Geometry: see drawing. Coordinates: mm, zero at the bounding-box minimum. A direction names the side the tool comes from. Coordinates: 2 decimals unless noted, no trailing zeros. Loops run counter-clockwise (first coordinate to the right, second up) from the corner with the lowest first, then second, coordinate; pieces in that order, holes last.
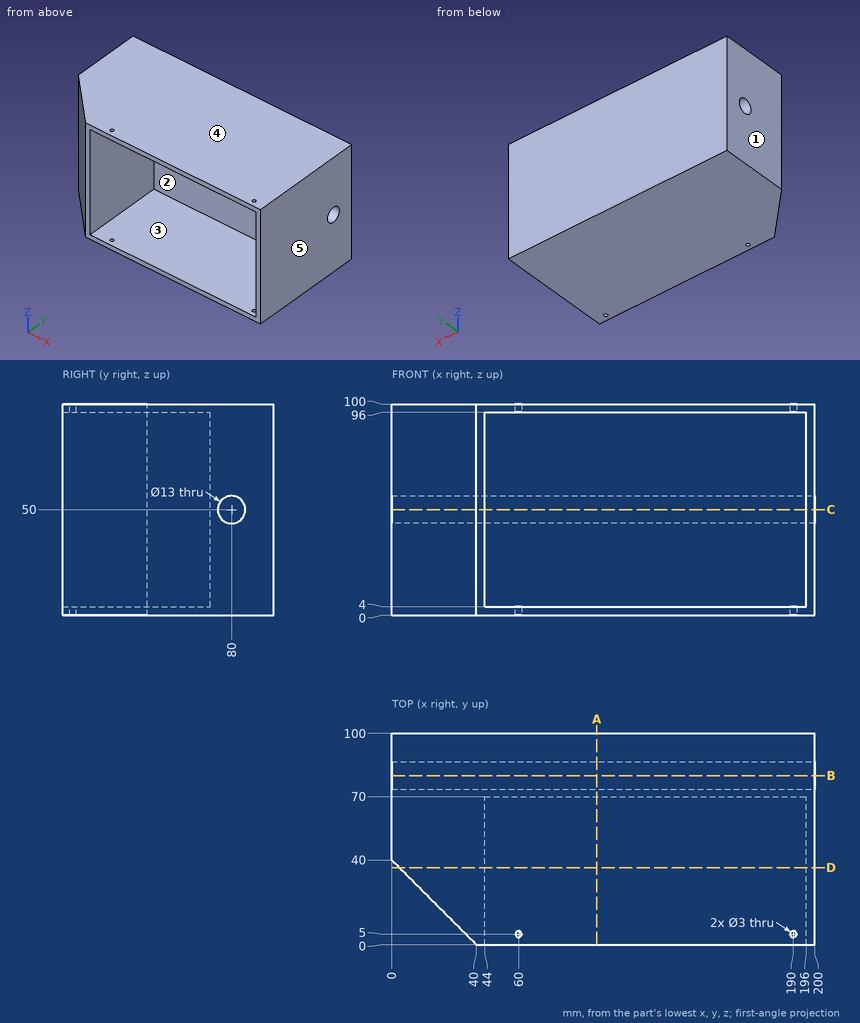
Item 1: Reachability of the marked faces 1 and 2 from +Z, -Z, +X, -X, +Y, -Y: full face, straight path, thin tool, end or side. Return the list, or none.
Result:
face 1: +Z, -Z, -X, +Y, -Y
face 2: -Y
Item 2: Section query A-A (x = 97). Output: boundary loops of the cut face in (y, z), then the cut area to 3 significant figures.
Result:
outline: (0, 0) - (100, 0) - (100, 100) - (0, 100) - (0, 96) - (70, 96) - (70, 4) - (0, 4) - close; hole circle Ø13 at (80, 50)
area: 3,430 mm2
Item 3: Line query: L1, parallel to Z at x = 54.5, y = 20.5; L2, parallel to X at y = 47.5, z = 79; L3, parallel to Y at x = 60, z = 98. Output: solid intervals per line, ascending.
Result:
L1: z = 0 to 4, 96 to 100
L2: x = 0 to 44, 196 to 200
L3: y = 0 to 3.5, 6.5 to 100
Item 4: Contact query for flat-ended pins moving along their axis: P1, Ø10, axis at y = 34.5, z = 59, coming from the -X side; P2, Ø3, axis at x = 147, z = 31.5, coming from the -Y side. Output: stop coordinate, or through.
Result:
P1: stops at x = 0.5
P2: stops at y = 70
Item 5: Mould query, pull axis X, two halves, no side actions, for the marked faces 3, 4 and 5. Classes: +X half, -X half, draft (parallel to the pull), parting line (faces both ways), or undercut.
Result:
face 3: undercut
face 4: draft
face 5: +X half
Item 6: Section query D-D (y = 36.5). Output: boundary loops of the cut face in (x, z), then the cut area to 3 significant figures.
Result:
outline: (3.5, 0) - (200, 0) - (200, 100) - (3.5, 100) - close; hole (44, 4) - (196, 4) - (196, 96) - (44, 96) - close
area: 5,670 mm2
Item 7: Section query B-B (y = 80). Output: boundary loops of the cut face in (x, z).
Result:
outline: (0, 0) - (200, 0) - (200, 43.5) - (0, 43.5) - close; (0, 56.5) - (200, 56.5) - (200, 100) - (0, 100) - close
Item 8: Section query C-C (z = 50). Output: boundary loops of the cut face in (x, y), then the cut area to 3 significant figures.
Result:
outline: (0, 40) - (40, 0) - (44, 0) - (44, 70) - (196, 70) - (196, 0) - (200, 0) - (200, 73.5) - (0, 73.5) - close; (0, 86.5) - (200, 86.5) - (200, 100) - (0, 100) - close
area: 5,960 mm2
